Could you check a few things on this model? Use its own coordinates, in mm. A direction names the side the tool comes from. Round coordinates to 2 decimals unless told otherwise and drop trailing zeros. Write each loop counter-clockwise with the first axis right and the second up, starting at its lowest first coordinate (ties: lowest second). Pieces come first, ordered by that corner, then holes. Notation, with made-up numbers: (8, 25) -> (12, 25) arc R28 cw to (12, 58) -> close; hole circle Ø4 at (49, 46.25). An arc over 180 degrees is marked (long way). Answer as CSV lines item,"result". Start each with the question number.
Q1. If I drill on line 1 (X direction, y = 549, z = 15.5); line 2 (X direction, y = 415, z = 14.25); line 3 (Y direction, x = 147, z = 15.5), over which ranges is the centre line in solid material (lowest first)? Write a range as [from, to].
Q2. For faces 1 (the flat face through (34, 516, 9)), 2 (the flat face through (43, 388, 18)), 3 (the flat face through (34, 596, 9)), 4 (the cylindrical face through (53.01, 322.85, 8.87)), which set-ups out of +Z, -Z, +X, -X, +Y, -Y let a thin tool reach every point of the face, with its end or its side?
Q3. Imagine slicing it at D-D on x = 75. Please give me the cut outline in (y, z).
Q4. Imagine slicing it at C-C on y = 570. Please give me the cut outline in (x, z), and give its area (3 significant figures).
Q5. If we mould it in two halves opening along Y, with no side actions, what happens to faces 5 (the flat face through (18, 605, 9)), 6 (the flat face through (34, 498, 9)), 7 (the cylindrical face through (3.919, 245.474, 8.874))? For each: pulls with the +Y half, pulls with the -Y half, needs draft (parallel to the pull), parting line crosses it, or undercut.
Q6. Imagine slicing it at A-A on z = 3.75. Please give me the cut outline in (x, y).
Q7. Will these pins go through, and if not, where does the flat tip stop? pin 1 Ø9 at (x, z) = (34, 4.5) entering from -Y; pin 2 Ø9 at (x, z) = (33.5, 7) entering from +Y; pin 3 Ø10 at (x, z) = (163.5, 16) entering from +Y.
Q8. Imagine slicing it at B-B on x = 32. Please give me the cut outline in (y, z).
from build123d import *

# Parameters (mm, degrees)
BOSS_EXTRU_1_DEPTH      = 18
ESQUISSE2_W             = 32
ESQUISSE2_H             = 18
ENL_V_MAT_EXTRU_1_DEPTH = 650.168699184
BOSS_EXTRU_2_DEPTH      = 18


with BuildPart() as part:
    # Esquisse1 → Boss.-Extru.1 (new body)
    with BuildSketch(Plane.XY):
        with BuildLine():
            Line((0, 614), (0, 253.412385947))
            ThreePointArc((0, 253.412385947), (4.022705111, 245.395407351), (12.854389163, 243.82841691))
            Line((12.854389163, 243.82841691), (202.854389163, 300.416030963))
            ThreePointArc((202.854389163, 300.416030963), (209.895445679, 311.442274181), (200, 320))
            Line((200, 320), (60, 320))
            ThreePointArc((60, 320), (52.928932188, 322.928932188), (50, 330))
            Line((50, 330), (50, 614))
            Line((50, 614), (0, 614))
        make_face()
    extrude(amount=BOSS_EXTRU_1_DEPTH)

    # Esquisse2 → Enlèv. mat.-Extru.1 (cut, through all)
    with BuildSketch(Plane.XY.offset(18)):
        with Locations((34, 605)):
            Rectangle(ESQUISSE2_W, ESQUISSE2_H)
        with Locations((34, 507)):
            Rectangle(ESQUISSE2_W, ESQUISSE2_H)
        with Locations((34, 409)):
            Rectangle(ESQUISSE2_W, ESQUISSE2_H)
    extrude(amount=-ENL_V_MAT_EXTRU_1_DEPTH, mode=Mode.SUBTRACT)

    # Esquisse3 → Boss.-Extru.2 (add)
    with BuildSketch(Plane.XY.offset(18)):
        with BuildLine():
            Line((208.660254038, 305), (213.660254038, 313.660254038))
            ThreePointArc((213.660254038, 313.660254038), (208.169872981, 334.150635095), (187.679491924, 328.660254038))
            Line((187.679491924, 328.660254038), (182.679491924, 320))
            Line((182.679491924, 320), (208.660254038, 305))
        make_face()
    extrude(amount=-BOSS_EXTRU_2_DEPTH)


solid = part.part
Checks:
1,line 1,"[0, 50]"
1,line 2,"[0, 18]"
1,line 3,"[283.78, 320]"
2,face 1,"+Z, -Z, +X"
2,face 2,"+Z, +X, -X, +Y, -Y"
2,face 3,"+Z, -Z, +X, +Y"
2,face 4,"+Z, -Z, +Y"
3,outline,"(262.34, 0) -> (320, 0) -> (320, 18) -> (262.34, 18) -> close"
4,outline,"(0, 0) -> (50, 0) -> (50, 18) -> (0, 18) -> close"
4,area,"900 mm^2"
5,face 5,"needs draft"
5,face 6,"undercut"
5,face 7,"pulls with the -Y half"
6,outline,"(0, 253.41) arc R10 ccw to (12.85, 243.83) -> (202.85, 300.42) arc R10 ccw to (208.66, 305) -> (213.66, 313.66) arc R15 ccw to (187.68, 328.66) -> (182.68, 320) -> (60, 320) arc R10 cw to (50, 330) -> (50, 400) -> (18, 400) -> (18, 418) -> (50, 418) -> (50, 498) -> (18, 498) -> (18, 516) -> (50, 516) -> (50, 596) -> (18, 596) -> (18, 614) -> (0, 614) -> close"
7,pin 1,"y = 248.79"
7,pin 2,"y = 596"
7,pin 3,"y = 320"
8,outline,"(249.53, 0) -> (400, 0) -> (400, 18) -> (249.53, 18) -> close; (418, 0) -> (498, 0) -> (498, 18) -> (418, 18) -> close; (516, 0) -> (596, 0) -> (596, 18) -> (516, 18) -> close"
